from build123d import *

# Parameters (mm, degrees)
F0_W     = 70
F0_H     = 70
F1_DEPTH = 1
F2_W     = 2
F2_H     = 12.7
F2_W_2   = 12.7
F2_H_2   = 2
F3_DEPTH = 2.001


with BuildPart() as f1:
    # F0 (on Front) → F1 (new body, symmetric)
    with BuildSketch(Plane.XZ):
        Rectangle(F0_W, F0_H)
    extrude(amount=F1_DEPTH, both=True)

    # F2 (on face) → F3 (cut, through all)
    with BuildSketch(Plane.XZ.offset(1)):
        with Locations((0, 26.11)):
            Rectangle(F2_W, F2_H)
        Polygon((-9.013975, 17.612662), (-15.363975, 28.611185), (-17.096025, 27.611185), (-10.746025, 16.612662), align=None)
        Polygon((-16.612662, 10.746025), (-27.611185, 17.096025), (-28.611185, 15.363975), (-17.612662, 9.013975), align=None)
        with Locations((-26.11, 0)):
            Rectangle(F2_W_2, F2_H_2)
        Polygon((-17.612662, -9.013975), (-28.611185, -15.363975), (-27.611185, -17.096025), (-16.612662, -10.746025), align=None)
        Polygon((-10.746025, -16.612662), (-17.096025, -27.611185), (-15.363975, -28.611185), (-9.013975, -17.612662), align=None)
        with Locations((0, -26.11)):
            Rectangle(F2_W, F2_H)
        Polygon((9.013975, -17.612662), (15.363975, -28.611185), (17.096025, -27.611185), (10.746025, -16.612662), align=None)
        Polygon((16.612662, -10.746025), (27.611185, -17.096025), (28.611185, -15.363975), (17.612662, -9.013975), align=None)
        with Locations((26.11, 0)):
            Rectangle(F2_W_2, F2_H_2)
        Polygon((17.612662, 9.013975), (28.611185, 15.363975), (27.611185, 17.096025), (16.612662, 10.746025), align=None)
        Polygon((10.746025, 16.612662), (17.096025, 27.611185), (15.363975, 28.611185), (9.013975, 17.612662), align=None)
    extrude(amount=-F3_DEPTH, mode=Mode.SUBTRACT)


solid = f1.part
Geometry check sheet. Reference: the model listing, model coordinates, mm. Round coordinates to 2 decimals unless told otherwise and drop trailing zeros. Order: outer loops, then holes, each group sorted by start corner. A loop starts at its lowest first (then second) coordinate and runs counter-clockwise, first axis right, second up. Notation, with made-up numbers: M -16,9.5 L 1,9.5 A20 cw 1,23.5 Z; hole C -38,-24 d4. An arc over 180 degrees is marked long. Write each question's results on one line, items separated by ' | '. Start each with the question number.
1. Cross-section at D-D on x = 25. Record the boundary of the cut face in (y, z).
2. Cross-section at A-A on z = -29.5. Record the boundary of the cut face in (x, y), plus the area to 3 significant figures.
3. Material ranges on L1, parallel to X at y = -0.3, z = -25; L2, parallel to Z at x = -18.5, y = -0.1; L3, parallel to X at y = 0, z = 9.5, recorded low to high. Write a range as from..to.
4. Cross-section at B-B on x = -14. Record the boundary of the cut face in (y, z).
5. Draft check along Z on faces 1 (the face through (0, 0, -35)), 2 (the face through (-22.035, -0.014, 13.877)), 3 (the face through (0, -1, 0)). Enter one of: pulls with the +Z half, pulls with the -Z half, needs draft (parallel to the pull), parting line crosses it, or undercut.
6. Cross-section at C-C on y = -0.6. Give the number of separate pieces and of enclosed holes in the cut face, plus the area to 3 significant figures.
Resolved:
1) outline: M -1,-35 L 1,-35 L 1,-15.59 L -1,-15.59 Z; M -1,-13.28 L 1,-13.28 L 1,-1 L -1,-1 Z; M -1,1 L 1,1 L 1,13.28 L -1,13.28 Z; M -1,15.59 L 1,15.59 L 1,35 L -1,35 Z
2) outline: M -35,-1 L -1,-1 L -1,1 L -35,1 Z; M 1,-1 L 35,-1 L 35,1 L 1,1 Z | area: 136 mm2
3) L1: -35..-15.59, -13.28..-1, 1..13.28, 15.59..35 | L2: -35..-11.84, -9.53..9.53, 11.84..35 | L3: -35..-18.45, -17.33..17.33, 18.45..35
4) outline: M -1,-35 L 1,-35 L 1,-26.25 L -1,-26.25 Z; M -1,-22.25 L 1,-22.25 L 1,22.25 L -1,22.25 Z; M -1,26.25 L 1,26.25 L 1,35 L -1,35 Z
5) face 1: pulls with the -Z half | face 2: undercut | face 3: needs draft
6) separate pieces: 1 | enclosed holes: 12 | area: 4,600 mm2
